Geometry check sheet. Reference: the model listing, model coordinates, mm. A direction names the side the tool comes from. Round coordinates to 2 decimals unless told otherwise and drop trailing zeros. Order: outer loops, then holes, each group sorted by start corner. A loop starts at its lowest first (then second) coordinate and runs counter-clockwise, first axis right, second up. Notation, with made-up numbers: (67, 83) -> (77, 83) arc R20 cw to (77, 116) -> close; hole circle Ø7 at (-1, 4.25). An arc over 180 degrees is marked (long way). Use a Markdown table: item, result. Add a question column.
Item 1: Sectioned sample at B-B, the plane y = 27. Record the cut outline in (x, z).
Item 2: Gauge pin test, flat ends, axial feed: pin 1 Ø14.5 at (x, z) = (0, 457.2) entering from +Y; pin 2 Ø18.5 at (x, z) = (0, 304.8) entering from +Y. Record the tip position at first contact, or that the pin passes through.
Item 3: Material ranges on probe 1 along X at (y, z) = (-37, 762); probe 2 along Y at (x, z) = (4, 111.5), recorded low to high. Write a range as [from, to].
Item 4: Set-up check for faces 1 (the cylindrical face through (1.72, 37.35, 93.85)), 2 (the flat face through (-36.576, -1, 451)): record each of +Z, -Z, +X, -X, +Y, -Y from which the full face is reachable in a straight line by a thin tool's end or side.
Item 5: Mould release check, pull along X, two halves, no side actions. Record for faces 3 (the cylindrical face through (-37.35, 6.3, 376.17)), 4 (the cylindrical face through (1.03, 37.35, 58.67)): pulls with the +X half, pulls with the -X half, needs draft (parallel to the pull), parting line crosses it, or undercut.
Item 6: Sectioned sample at A-A, the plane z = 254. Record the cut outline in (x, y).
from build123d import *

# Parameters (mm, degrees)
F0_W       = 76.2
F0_H       = 76.2
F0_W_2     = 73.152
F0_H_2     = 73.152
F1_DEPTH   = 914.4
F6_D       = 15.875
F6_ON_F3_D = 15.875


with BuildPart() as f1:
    # F0 (on Top) → F1 (new body)
    with BuildSketch(Plane.XY):
        Rectangle(F0_W, F0_H)
        Rectangle(F0_W_2, F0_H_2, mode=Mode.SUBTRACT)
    extrude(amount=F1_DEPTH)

    # F6 (through all)
    with Locations(Plane.YZ.offset(76.2)):
        with Locations((0, 25.4), (0, 76.2), (0, 127), (0, 177.8), (0, 228.6), (0, 279.4), (0, 330.2), (0, 381), (0, 431.8), (0, 482.6), (0, 533.4), (0, 584.2), (0, 635), (0, 685.8), (0, 736.6), (0, 787.4), (0, 838.2), (0, 889)):
            Hole(F6_D / 2)

    # F6 on F3 (through all)
    with Locations(Plane.XZ.offset(76.2)):
        with Locations((0, 863.6), (0, 812.8), (0, 762), (0, 711.2), (0, 660.4), (0, 609.6), (0, 558.8), (0, 508), (0, 457.2), (0, 406.4), (0, 355.6), (0, 304.8), (0, 254), (0, 203.2), (0, 152.4), (0, 101.6), (0, 50.8)):
            Hole(F6_ON_F3_D / 2)


solid = f1.part
Found:
| question | item | result |
|---|---|---|
| 1 | outline | (-38.1, 0) -> (-36.58, 0) -> (-36.58, 914.4) -> (-38.1, 914.4) -> close; (36.58, 0) -> (38.1, 0) -> (38.1, 914.4) -> (36.58, 914.4) -> close |
| 2 | pin 1 | passes through |
| 2 | pin 2 | stops at y = 38.1 |
| 3 | probe 1 | x = [-38.1, -7.94], [7.94, 38.1] |
| 3 | probe 2 | y = [-38.1, -36.58], [36.58, 38.1] |
| 4 | face 1 | +Y, -Y |
| 4 | face 2 | +Z, -Z |
| 5 | face 3 | needs draft |
| 5 | face 4 | undercut |
| 6 | outline | (-38.1, -38.1) -> (-7.94, -38.1) -> (-7.94, -36.58) -> (-36.58, -36.58) -> (-36.58, 36.58) -> (-7.94, 36.58) -> (-7.94, 38.1) -> (-38.1, 38.1) -> close; (7.94, -38.1) -> (38.1, -38.1) -> (38.1, 38.1) -> (7.94, 38.1) -> (7.94, 36.58) -> (36.58, 36.58) -> (36.58, -36.58) -> (7.94, -36.58) -> close |
